Read the model definition and answer for the solid it produces. Units are mm, in the model's axes. A direction names the side the tool comes from. Give positions to 0.01 mm unless a question says otherwise; leave off trailing zeros. Write each loop counter-clockwise with the first axis right and the second up, starting at its lowest first coordinate (ties: lowest second). Pieces come first, ordered by that corner, then holes. Notation, with made-up numbers: (-31.75, 87) - (8.25, 87) arc R15 cw to (8.25, 98) - close; hole circle Ø8 at (25, 56.5). An arc over 180 degrees is marked (long way). Use CSV: the item, a comma, the result in double quotes. Start each with the question number.
from build123d import *


with BuildPart() as f1:
    # F0 (on Front) → F1 (revolve)
    with BuildSketch(Plane.XZ):
        with BuildLine():
            Line((-177.8, 0), (0, 0))
            Line((0, 0), (0, 0.254))
            Line((0, 0.254), (-177.994901, 0.254))
            ThreePointArc((-177.994901, 0.254), (-181.860536, -1.058206), (-184.12853, -4.452499))
            Line((-184.12853, -4.452499), (-186.338441, -12.7))
            Line((-186.338441, -12.7), (-190.910441, -12.7))
            Line((-190.910441, -12.7), (-190.910441, -20.32))
            Line((-190.910441, -20.32), (-184.560441, -20.32))
            Line((-184.560441, -20.32), (-184.560441, -12.7))
            Line((-184.560441, -12.7), (-186.075481, -12.7))
            Line((-186.075481, -12.7), (-183.933629, -4.706499))
            ThreePointArc((-183.933629, -4.706499), (-181.665635, -1.312206), (-177.8, 0))
        make_face()
    revolve(axis=Axis((0, 0, -46.123708), (0, 0, -1)))


solid = f1.part
(1) For a pull along Z with two mould halves and no side action, classify faces 1 (the face through (-175.539, 55.28, -5.095)), 2 (the face through (2, 2, 0)), 3 (the face through (39.945, -179.885, -4.968)), 4 (the face through (-176.038, 55.437, -16.457)) as pulls with the +Z half, pulls with the -Z half, needs draft (parallel to the pull), parting line crosses it, or undercut.
(2) Consider probe 1 along X at (y, z) = (-4, -5); probe 2 along Y at (x, z) = (0, -15.75); probe 3 along Z at (x, y) = (-133.5, -21). Determine where each line is inside the solid, lowest interval first.
(3) Given P1, Ø4, axis at x = -96, z = -14, coming from the -Y side; P2, Ø4, axis at x = -74.5, y = -97, coming from the -Z side; P3, Ø3, axis at y = 83, z = -9, coming from the +X side, each flat-ended and moving along its own axis, determine where each tip first touches the part or whether it passes through.
(4) Which of the six approach directions +Z, -Z, +X, -X, +Y, -Y give full straight-line access (tool end or side, diameter ignored) to faces 5 (the face through (42, -183, -12.7)), 6 (the face through (-2, 2, 0.254))?
(5) The part is cut by section A-A on y = 0. Write down the section's boundary in (x, z), plus the area to 3 significant figures.
Reported:
1,face 1,"undercut"
1,face 2,"pulls with the -Z half"
1,face 3,"pulls with the +Z half"
1,face 4,"needs draft"
2,probe 1,"-184.23 to -183.97, 183.97 to 184.23"
2,probe 2,"-190.91 to -184.56, 184.56 to 190.91"
2,probe 3,"0 to 0.25"
3,P1,"y = -166.16"
3,P2,"z = 0"
3,P3,"x = 166.59"
4,face 5,"+Z"
4,face 6,"+Z, +X, -X, +Y, -Y"
5,outline,"(-190.91, -20.32) - (-184.56, -20.32) - (-184.56, -12.7) - (-186.08, -12.7) - (-183.93, -4.71) arc R6.35 cw to (-177.8, 0) - (177.8, 0) arc R6.35 cw to (183.93, -4.71) - (186.08, -12.7) - (184.56, -12.7) - (184.56, -20.32) - (190.91, -20.32) - (190.91, -12.7) - (186.34, -12.7) - (184.13, -4.45) arc R6.35 ccw to (177.99, 0.25) - (-177.99, 0.25) arc R6.35 ccw to (-184.13, -4.45) - (-186.34, -12.7) - (-190.91, -12.7) - close"
5,area,"196 mm²"
